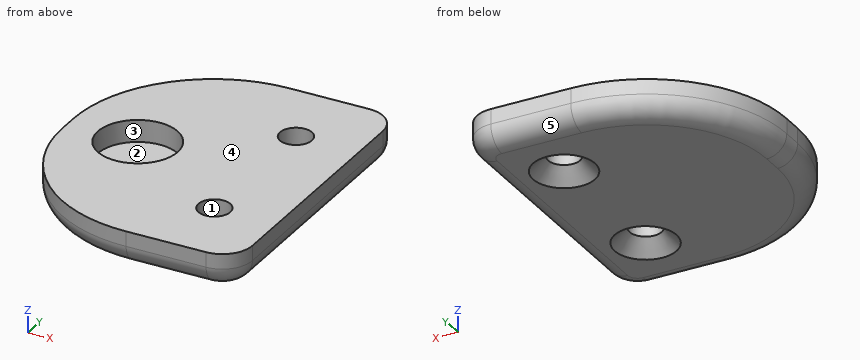
```python
from build123d import *

# Parameters (mm, degrees)
SKETCH_1_R          = 1.6
EXTRUDE_1_DEPTH     = 3.5
SKETCH_2_R          = 4
CUT_EXTRUDE_1_DEPTH = 2.2
FILLET_1_R          = 2
CHAMFER_1_SIZE      = 1.5


with BuildPart() as part:
    # Эскиз1 → Бобышка-Вытянуть1 (new body)
    with BuildSketch(Plane.XY):
        with BuildLine():
            Line((1.5, 15), (9.5, 15))
            ThreePointArc((9.5, 15), (11.621320344, 14.121320344), (12.5, 12))
            Line((12.5, 12), (12.5, -12))
            ThreePointArc((12.5, -12), (11.621320344, -14.121320344), (9.5, -15))
            Line((9.5, -15), (1.5, -15))
            ThreePointArc((1.5, -15), (-8.399494937, -10.899494937), (-12.5, -1))
            Line((-12.5, -1), (-12.5, 1))
            ThreePointArc((-12.5, 1), (-8.399494937, 10.899494937), (1.5, 15))
        make_face()
        with Locations((6.25, 7.5)):
            Circle(SKETCH_1_R, mode=Mode.SUBTRACT)
        with Locations((6.25, -7.5)):
            Circle(SKETCH_1_R, mode=Mode.SUBTRACT)
    extrude(amount=EXTRUDE_1_DEPTH)

    # Эскиз2 → Вырез-Вытянуть1 (cut)
    with BuildSketch(Plane.XY.offset(3.5)):
        with Locations((-5.5, 0)):
            Circle(SKETCH_2_R)
    extrude(amount=-CUT_EXTRUDE_1_DEPTH, mode=Mode.SUBTRACT)

    # Скругление1
    fillet_1_edges = [part.edges().sort_by_distance(p)[0] for p in [
        (12.5, 0, 0),
        (11.621320344, -14.121320344, 0),
        (5.5, -15, 0),
        (-8.399494937, -10.899494937, 0),
        (-12.5, 0, 0),
        (-8.399494937, 10.899494937, 0),
        (5.5, 15, 0),
        (11.621320344, 14.121320344, 0),
    ]]
    fillet(fillet_1_edges, radius=FILLET_1_R)

    # Фаска1
    chamfer_1_edges = [part.edges().sort_by_distance(p)[0] for p in [
        (4.65, 7.5, 0),
        (4.65, -7.5, 0),
    ]]
    chamfer(chamfer_1_edges, length=CHAMFER_1_SIZE)


solid = part.part
```
Work out the finished part from the listing and answer in its coordinate system (mm). Face numbers are marked on the shaded views. A direction names the side the tool comes from. Round coordinates to 2 decimals unless told otherwise and drop trailing zeros. Loops run counter-clockwise (first coordinate to the right, second up) from the corner with the lowest first, then second, coordinate; pieces in that order, holes last. Notation, with made-up numbers: M 69.5,-32.75 L 126.5,-32.75 A27 ccw 126.5,-6.75 Z; hole C -33.75,64.25 d10. An arc over 180 degrees is marked long. Use CSV: the item, a comma, the result in double quotes.
Q1. A tool of negligible diameter and unlimited length cuts with its end or side. For the marked faces 1 and 2, from which of +Z, -Z, +X, -X, +Y, -Y can it reach the whole face along a straight path? Write none if from no direction.
Determined:
face 1,"+Z, -Z"
face 2,"+Z"
Q2. Consider L1, parallel to Y at x = 6.25, z = 2.5; L2, parallel to Y at x = 5.25, z = 0.6; L3, parallel to X at y = -6.5, z = 1.1. Determine where each line is inside the solid, lowest interval first.
Determined:
L1,"-15 to -9.1, -5.9 to 5.9, 9.1 to 15"
L2,"-14.43 to -9.79, -5.21 to 5.21, 9.79 to 14.43"
L3,"-11.14 to 4.52, 7.98 to 12.29"
Q3. Section B-B, the plane z = 3 is taken. Determine the outline of the cut face in (x, y), then the cut area to 3 significant figures.
Determined:
outline,"M -12.5,-1 A14 ccw 1.5,-15 L 9.5,-15 A3 ccw 12.5,-12 L 12.5,12 A3 ccw 9.5,15 L 1.5,15 A14 ccw -12.5,1 Z; hole C -5.5,0 d8; hole C 6.25,-7.5 d3.2; hole C 6.25,7.5 d3.2"
area,"596 mm2"
Q4. Section C-C, the plane z = 0.9 is taken. State how many separate pieces and enclosed holes the cut face has, then the cut area to 3 significant figures.
Determined:
separate pieces,"1"
enclosed holes,"2"
area,"600 mm2"
Q5. Section A-A, the plane x = 6.25 is taken. Determine the outline of the cut face in (y, z).
Determined:
outline,"M -15,2 A2 ccw -13,0 L -10.6,0 L -9.1,1.5 L -9.1,3.5 L -15,3.5 Z; M -5.9,1.5 L -4.4,0 L 4.4,0 L 5.9,1.5 L 5.9,3.5 L -5.9,3.5 Z; M 9.1,1.5 L 10.6,0 L 13,0 A2 ccw 15,2 L 15,3.5 L 9.1,3.5 Z"
Q6. The mould has two halves that part along Y. Classify the marked faces 3, 4 and 5: pulls with the +Y half, pulls with the -Y half, needs draft (parallel to the pull), parting line crosses it, or undercut.
Determined:
face 3,"undercut"
face 4,"needs draft"
face 5,"pulls with the +Y half"
Q7. Each of these flat-tipped pins is pushed along its axis until it touches: pin 1 (1 mm diameter, centred on x = -6, z = 3, fed in from -Y); pin 2 (3.5 mm diameter, centred on x = 6.25, y = -7.5, fed in from -Z); pin 3 (5 mm diameter, centred on x = -5.5, y = 0, fed in from +Z); pin 4 (1.9 mm diameter, centred on x = 6.25, y = 7.5, fed in from +Z). Where does it stop, or does it pass through?
Determined:
pin 1,"y = -13.12"
pin 2,"z = 1.35"
pin 3,"z = 1.3"
pin 4,"through"
